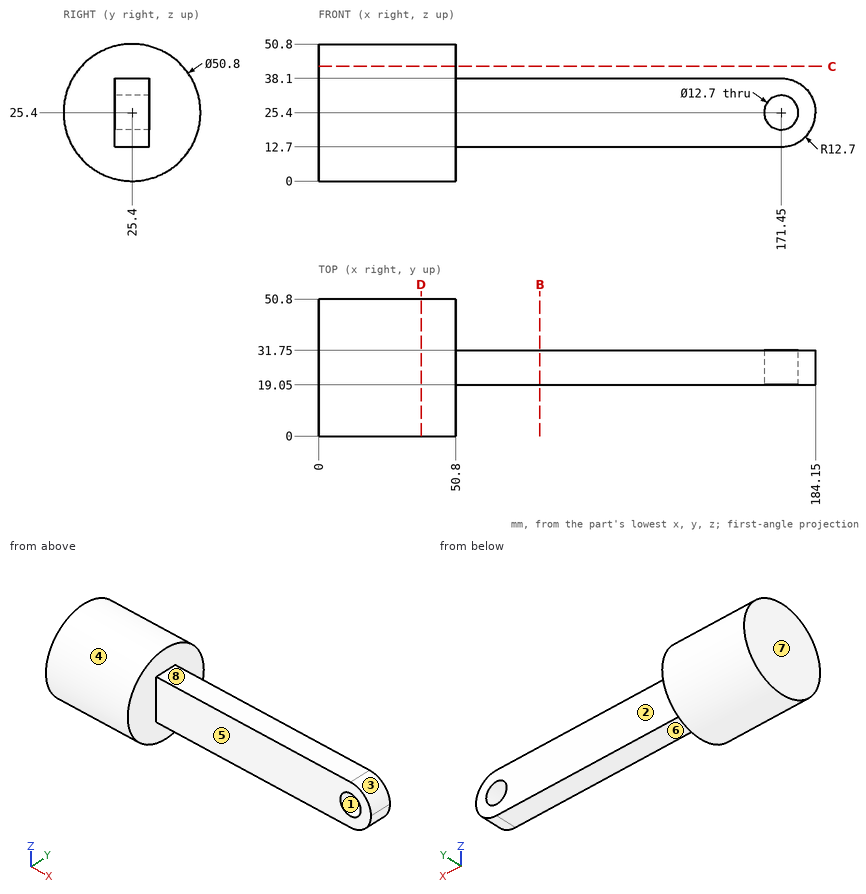
Study the drawing (mm; zero at the part's minimum x, y, z) and answer. A direction names the side the tool comes from. Give positions to 0.01 mm unless a question says otherwise; leave off trailing zeros. Loops run counter-clockwise (first coordinate to the right, second up) from the corner with the lowest first, then second, coordinate; pieces in that order, holes last. Notation, with made-up numbers: M 52.5,-33 L 94.5,-33 A7 cw 94.5,-26 Z; hole C 23,73 d6. An arc over 180 degrees is marked long. One line per item, written item: value. Start each with the question number.
1. Find the intervals of material crossed by probe 1 along Z at (x, y) = (171, 27); probe 2 along X at (y, z) = (28, 25); probe 3 along X at (y, z) = (16, 7), in increasing order.
2. Find section D-D (x = 38). Give the vertices of the cut face in (y, z).
3. Each of these flat-tipped pins is pushed along its axis until it touches: P1, Ø3, axis at x = 128, z = 17, coming from the +Y side; P2, Ø4, axis at x = 134.5, y = 25, coming from the +Z side; P3, Ø1, axis at y = 43.5, z = 42, coming from the +X side; P4, Ø7.5, axis at x = 171.45, z = 25.4, coming from the +Y side. Where does it stop, or does it pass through?
4. Determine the mould class of the marked faces 1, 2 and 3 for opening direction X: released by +X, released by -X, zero draft, split by the parting line, or undercut.
5. Find section B-B (x = 82). Give the vertices of the cut face in (y, z), and give its area (3 significant figures).
6. Find section C-C (z = 42.5). Give the vertices of the cut face in (x, y).
7. Which of the six approach directions +Z, -Z, +X, -X, +Y, -Y give full straight-line access (tool end or side, diameter ignored) to the marked faces 4, 5, 6, 7 and 8?
Reported:
1. probe 1: z = 12.7 to 19.07, 31.73 to 38.1
1. probe 2: x = 0 to 165.11, 177.79 to 184.14
1. probe 3: x = 0 to 50.8
2. outline: C 25.4,25.4 d50.8
3. P1: stops at y = 31.75
3. P2: stops at z = 38.1
3. P3: stops at x = 50.8
3. P4: passes through
4. face 1: undercut
4. face 2: zero draft
4. face 3: released by +X
5. outline: M 19.05,12.7 L 31.75,12.7 L 31.75,38.1 L 19.05,38.1 Z
5. area: 323 mm²
6. outline: M 0,6.62 L 50.8,6.62 L 50.8,44.18 L 0,44.18 Z
7. face 4: +X, -X
7. face 5: +Z, -Z, +X, -Y
7. face 6: -Z, +X, +Y, -Y
7. face 7: +Z, -Z, -X, +Y, -Y
7. face 8: +Z, +X, +Y, -Y
